Source: CAD feature listing. Evaluate the final solid. Frame: model axes, mm. A direction names the side the tool comes from. Give positions to 0.01 mm unless a question says otherwise; leave off trailing zeros. Loops run counter-clockwise (first coordinate to the right, second up) from the corner with the lowest first, then second, coordinate; pieces in that order, holes last. Notation, with made-up numbers: (59.5, 70) -> (87.5, 70) arc R24 cw to (87.5, 90) -> close; hole circle Ø1 at (-31, 57.5). An arc over 180 degrees is marked (long way). Put each result on its own line as item: value.
```python
from build123d import *

# Parameters (mm, degrees)
EXTRUDE2_DEPTH = 6.35


with BuildPart() as part:
    # Sketch1 → Extrude2 (new body)
    with BuildSketch(Plane.XY):
        Polygon((47.660264722, 0), (76.2, 0), (76.2, 6.35), (82.55, 6.35), (82.55, 0), (92.202, 0), (92.202, 6.35), (98.552, 6.35), (98.552, 0), (320.548, 0), (320.548, 6.35), (326.898, 6.35), (326.898, 0), (336.55, 0), (336.55, 6.35), (342.9, 6.35), (342.9, 0), (371.439735278, 0), (419.1, 82.55), (387.35, 82.55), (387.35, 88.9), (361.95, 88.9), (361.95, 82.55), (311.15, 82.55), (311.15, 88.9), (285.75, 88.9), (285.75, 82.55), (276.225, 82.55), (276.225, 41.275), (269.875, 41.275), (269.875, 82.55), (149.225, 82.55), (149.225, 41.275), (142.875, 41.275), (142.875, 82.55), (133.35, 82.55), (133.35, 88.9), (107.95, 88.9), (107.95, 82.55), (57.15, 82.55), (57.15, 88.9), (31.75, 88.9), (31.75, 82.55), (0, 82.55), align=None)
        with BuildLine():
            Line((155.575, 67.749415869), (155.575, 14.800584131))
            ThreePointArc((155.575, 14.800584131), (156.901171335, 12.56939163), (159.494858247, 12.668075931))
            Line((159.494858247, 12.668075931), (200.40986459, 39.142491801))
            ThreePointArc((200.40986459, 39.142491801), (201.570006344, 41.275), (200.40986459, 43.407508199))
            Line((200.40986459, 43.407508199), (159.494858247, 69.881924069))
            ThreePointArc((159.494858247, 69.881924069), (156.901171335, 69.98060837), (155.575, 67.749415869))
        make_face(mode=Mode.SUBTRACT)
        with BuildLine():
            Line((170.020448202, 6.35), (249.079551798, 6.35))
            ThreePointArc((249.079551798, 6.35), (251.515549625, 8.170615133), (250.459410045, 11.022508199))
            Line((250.459410045, 11.022508199), (209.55, 37.493302934))
            Line((209.55, 37.493302934), (168.640589955, 11.022508199))
            ThreePointArc((168.640589955, 11.022508199), (167.584450375, 8.170615133), (170.020448202, 6.35))
        make_face(mode=Mode.SUBTRACT)
        with BuildLine():
            Line((52.031551003, 11.033734326), (77.262001053, 31.718906867))
            ThreePointArc((77.262001053, 31.718906867), (78.181456091, 33.910104112), (76.886676101, 35.902662194))
            Line((76.886676101, 35.902662194), (22.118136541, 66.378961445))
            ThreePointArc((22.118136541, 66.378961445), (19.07288135, 65.941246674), (18.683371551, 62.889451217))
            Line((18.683371551, 62.889451217), (48.221461062, 11.727979426))
            ThreePointArc((48.221461062, 11.727979426), (49.965843374, 10.499123351), (52.031551003, 11.033734326))
        make_face(mode=Mode.SUBTRACT)
        with BuildLine():
            Line((61.828236325, 10.8542451), (84.780365617, 29.671537445))
            ThreePointArc((84.780365617, 29.671537445), (86.163798888, 30.2371328), (87.625811497, 29.926802573))
            Line((87.625811497, 29.926802573), (121.442109591, 11.109510228))
            ThreePointArc((121.442109591, 11.109510228), (122.665621474, 8.252017233), (120.207049127, 6.35))
            Line((120.207049127, 6.35), (104.902, 6.35))
            Line((104.902, 6.35), (104.902, 12.7))
            Line((104.902, 12.7), (69.85, 12.7))
            Line((69.85, 12.7), (69.85, 6.35))
            Line((69.85, 6.35), (63.438621741, 6.35))
            ThreePointArc((63.438621741, 6.35), (61.046887793, 8.034892566), (61.828236325, 10.8542451))
        make_face(mode=Mode.SUBTRACT)
        with BuildLine():
            Line((26.081413037, 71.440489772), (83.920586204, 39.255517086))
            ThreePointArc((83.920586204, 39.255517086), (85.382598814, 38.945186859), (86.766032084, 39.510782213))
            Line((86.766032084, 39.510782213), (126.023202606, 71.6957549))
            ThreePointArc((126.023202606, 71.6957549), (126.804551138, 74.515107434), (124.41281719, 76.2))
            Line((124.41281719, 76.2), (27.316473501, 76.2))
            ThreePointArc((27.316473501, 76.2), (24.857901154, 74.297982767), (26.081413037, 71.440489772))
        make_face(mode=Mode.SUBTRACT)
        with BuildLine():
            Line((94.284396649, 37.463412792), (132.374614584, 68.691659953))
            ThreePointArc((132.374614584, 68.691659953), (135.071559028, 69.023278411), (136.525, 66.727414853))
            Line((136.525, 66.727414853), (136.525, 14.303625696))
            ThreePointArc((136.525, 14.303625696), (135.272351238, 12.114030576), (132.749939536, 12.084115469))
            Line((132.749939536, 12.084115469), (94.659721601, 33.279657465))
            ThreePointArc((94.659721601, 33.279657465), (93.364941611, 35.272215547), (94.284396649, 37.463412792))
        make_face(mode=Mode.SUBTRACT)
        with BuildLine():
            Line((168.640589955, 71.527491801), (209.55, 45.056697066))
            Line((209.55, 45.056697066), (250.459410045, 71.527491801))
            ThreePointArc((250.459410045, 71.527491801), (251.515549625, 74.379384867), (249.079551798, 76.2))
            Line((249.079551798, 76.2), (170.020448202, 76.2))
            ThreePointArc((170.020448202, 76.2), (167.584450375, 74.379384867), (168.640589955, 71.527491801))
        make_face(mode=Mode.SUBTRACT)
        with BuildLine():
            Line((282.575, 66.727414853), (282.575, 14.303625696))
            ThreePointArc((282.575, 14.303625696), (283.827648762, 12.114030576), (286.350060464, 12.084115469))
            Line((286.350060464, 12.084115469), (324.440278399, 33.279657465))
            ThreePointArc((324.440278399, 33.279657465), (325.735058389, 35.272215547), (324.815603351, 37.463412792))
            Line((324.815603351, 37.463412792), (286.725385416, 68.691659953))
            ThreePointArc((286.725385416, 68.691659953), (284.028440972, 69.023278411), (282.575, 66.727414853))
        make_face(mode=Mode.SUBTRACT)
        with BuildLine():
            Line((391.783526499, 76.2), (294.68718281, 76.2))
            ThreePointArc((294.68718281, 76.2), (292.295448862, 74.515107434), (293.076797394, 71.6957549))
            Line((293.076797394, 71.6957549), (332.333967916, 39.510782213))
            ThreePointArc((332.333967916, 39.510782213), (333.717401186, 38.945186859), (335.179413796, 39.255517086))
            Line((335.179413796, 39.255517086), (393.018586963, 71.440489772))
            ThreePointArc((393.018586963, 71.440489772), (394.242098846, 74.297982767), (391.783526499, 76.2))
        make_face(mode=Mode.SUBTRACT)
        with BuildLine():
            Line((314.198, 12.7), (314.198, 6.35))
            Line((314.198, 6.35), (298.892950873, 6.35))
            ThreePointArc((298.892950873, 6.35), (296.434378526, 8.252017233), (297.657890409, 11.109510228))
            Line((297.657890409, 11.109510228), (331.474188503, 29.926802573))
            ThreePointArc((331.474188503, 29.926802573), (332.936201112, 30.2371328), (334.319634383, 29.671537445))
            Line((334.319634383, 29.671537445), (357.271763675, 10.8542451))
            ThreePointArc((357.271763675, 10.8542451), (358.053112207, 8.034892566), (355.661378259, 6.35))
            Line((355.661378259, 6.35), (349.25, 6.35))
            Line((349.25, 6.35), (349.25, 12.7))
            Line((349.25, 12.7), (314.198, 12.7))
        make_face(mode=Mode.SUBTRACT)
        with BuildLine():
            Line((400.416628449, 62.889451217), (370.878538938, 11.727979426))
            ThreePointArc((370.878538938, 11.727979426), (369.134156626, 10.499123351), (367.068448997, 11.033734326))
            Line((367.068448997, 11.033734326), (341.837998947, 31.718906867))
            ThreePointArc((341.837998947, 31.718906867), (340.918543909, 33.910104112), (342.213323899, 35.902662194))
            Line((342.213323899, 35.902662194), (396.981863459, 66.378961445))
            ThreePointArc((396.981863459, 66.378961445), (400.02711865, 65.941246674), (400.416628449, 62.889451217))
        make_face(mode=Mode.SUBTRACT)
        with BuildLine():
            Line((259.605141753, 12.668075931), (218.69013541, 39.142491801))
            ThreePointArc((218.69013541, 39.142491801), (217.529993656, 41.275), (218.69013541, 43.407508199))
            Line((218.69013541, 43.407508199), (259.605141753, 69.881924069))
            ThreePointArc((259.605141753, 69.881924069), (262.198828665, 69.98060837), (263.525, 67.749415869))
            Line((263.525, 67.749415869), (263.525, 14.800584131))
            ThreePointArc((263.525, 14.800584131), (262.198828665, 12.56939163), (259.605141753, 12.668075931))
        make_face(mode=Mode.SUBTRACT)
    extrude(amount=EXTRUDE2_DEPTH)


solid = part.part
```
(1) Section C-C on x = 112. Return loops of the section in (y, z), then the cut area to 3 significant figures.
Calculated:
outline: (0, 0) -> (6.35, 0) -> (6.35, 6.35) -> (0, 6.35) -> close; (16.36, 0) -> (23.63, 0) -> (23.63, 6.35) -> (16.36, 6.35) -> close; (51.99, 0) -> (60.2, 0) -> (60.2, 6.35) -> (51.99, 6.35) -> close; (76.2, 0) -> (88.9, 0) -> (88.9, 6.35) -> (76.2, 6.35) -> close
area: 219 mm²
(2) First-contact query: P1, Ø1.9, axis at x = 138.5, z = 2, coming from the +Y side; P2, Ø1.9, axis at x = 95.5, z = 4, coming from the -Y side; P3, Ø3, axis at y = 63, z = 3, coming from the +X side. Flat tips, straight axial feed; report the tip coordinate or a pass-through.
Calculated:
P1: stops at y = 82.55
P2: stops at y = 6.35
P3: stops at x = 408.68
(3) Reachability of faces 1 (the flat face through (394.94, 40.7, 3.13)), 2 (the flat face through (106.12, 55.38, 3.13)) from +Z, -Z, +X, -X, +Y, -Y: full face, straight path, thin tool, end or side. Return the list, or none.
Calculated:
face 1: +Z, -Z, +X, -Y
face 2: +Z, -Z
(4) Section B-B on z = 2.5. Give the number of separate pieces and of enclosed holes in the cut face, then the cut area to 3 significant figures.
Calculated:
separate pieces: 1
enclosed holes: 12
area: 13,700 mm²
(5) Line query: probe 1 along X at (y, z) = (72, 2.5) (3 decimals); probe 2 along Y at (x, z) = (331, 3.5); probe 3 along Y at (x, z) = (285, 5.5). Output: solid intervals per line, ascending. Write a range as from..to.
Calculated:
probe 1: x = 6.091..25.394, 126.335..142.875, 149.225..168.098, 251.002..269.875, 276.225..292.765, 393.706..413.009
probe 2: y = 0..12.7, 29.66..40.6, 76.2..82.55
probe 3: y = 0..11.77, 69.26..82.55
(6) Draft query along X for faces 3 (the flat face through (23.5, 41.85, 3.13)), 4 (the flat face through (209, 41, 6.35)), 5 (the flat face through (179.666, 25.72, 3.131)). Return one class per face: released by +X, released by -X, zero draft, split by the parting line, or undercut.
Calculated:
face 3: released by -X
face 4: zero draft
face 5: undercut
(7) Section A-A on x = 224.5. Return loops of the section in (y, z).
Calculated:
outline: (0, 0) -> (6.35, 0) -> (6.35, 6.35) -> (0, 6.35) -> close; (27.82, 0) -> (35.38, 0) -> (35.38, 6.35) -> (27.82, 6.35) -> close; (47.17, 0) -> (54.73, 0) -> (54.73, 6.35) -> (47.17, 6.35) -> close; (76.2, 0) -> (82.55, 0) -> (82.55, 6.35) -> (76.2, 6.35) -> close
